For this review, use the dimensioned drawing (mm, ordinates from the lowest corner) and the shaded views. A direction names the side the tool comes from. Coordinates: 2 decimals unless noted, no trailing zeros. Loops run counter-clockwise (first coordinate to the right, second up) from the corner with the lowest first, then second, coordinate; pieces in that order, holes last. Notation, with made-up numbers: (73.25, -1) - (132.25, -1) arc R16 ccw to (132.25, 16) - close; hole circle Ø6 at (43.5, 32). An arc over 180 degrees is marked (long way). One line per item, written item: value. Start each with the question number.
1. We need section A-A, the plane z = 12. Give the boundary of the cut face in (x, y).
2. We need section D-D, the plane y = 12. Give the boundary of the cut face in (x, z).
3. For the marked faces 4 and 5, list the 3-axis set-ups (+Z, -Z, +X, -X, +Y, -Y) from which the entire face can be reached by the end or side of a thin tool; tool diameter is ignored.
4. Mouldability with a two-part tool opening along Y and no side actions: class the marked faces 1, 2 and 3 as +Y half, -Y half, draft (parallel to the pull), parting line (faces both ways), or undercut.
5. We need section C-C, the plane x = 8. Give the boundary of the cut face in (y, z), then the cut area to 3 significant figures.
6. Insertion check: P1, Ø7, axis at y = 23, z = 14, coming from the -X side; P2, Ø2, axis at y = 23.5, z = 4, coming from the -X side; P3, Ø7.5, axis at x = 20.5, y = 13.5, coming from the +Z side; P4, Ø8, axis at y = 12.5, z = 15.5, coming from the +X side. Each pin has a flat end and moves straight along its axis. Give the tip position at first contact, or say it passes through.
7. To check wall thickness, follow line 1 (X direction, y = 32, z = 21.5); line 2 (Z direction, x = 19.5, y = 13); line 3 (X direction, y = 27, z = 4.5). State the ranges of each line that lie inside material, in increasing order.
8. We need section B-B, the plane y = 24.5. Give the boundary of the cut face in (x, z).
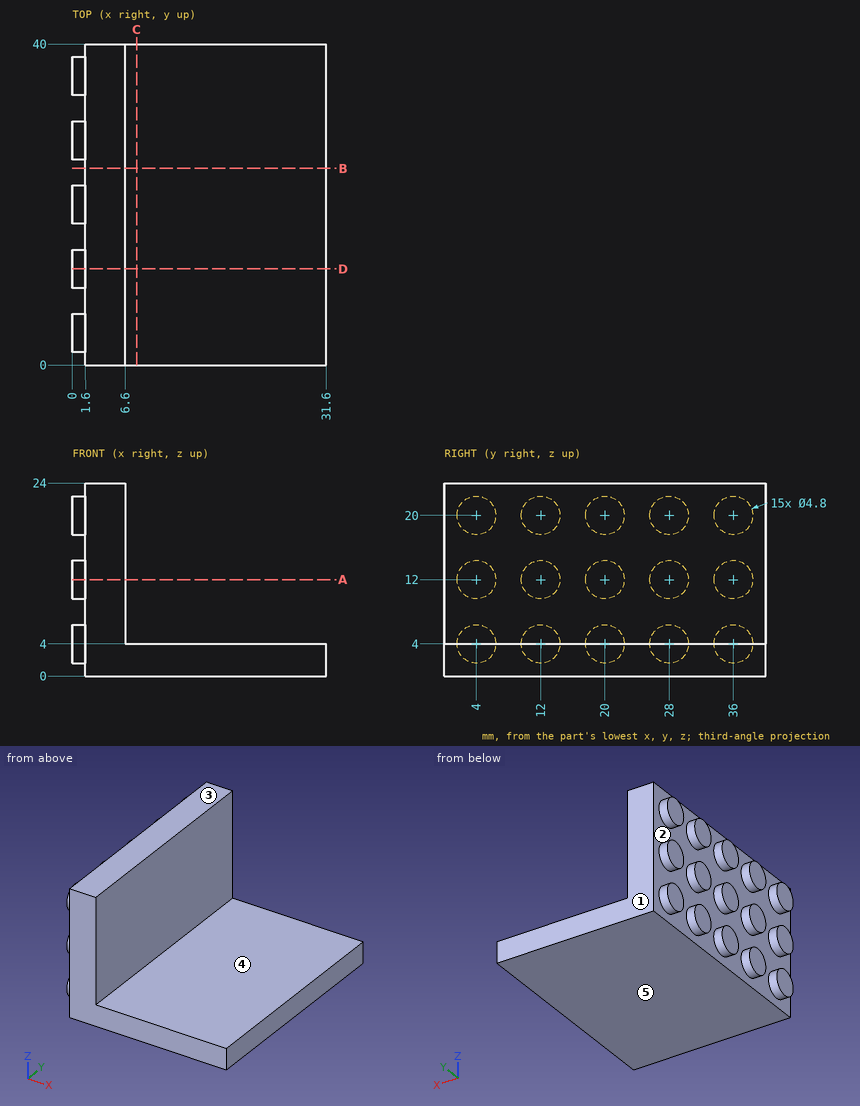
Findings below:
1. outline: (0, 1.6) - (1.6, 1.6) - (1.6, 0) - (6.6, 0) - (6.6, 40) - (1.6, 40) - (1.6, 38.4) - (0, 38.4) - (0, 33.6) - (1.6, 33.6) - (1.6, 30.4) - (0, 30.4) - (0, 25.6) - (1.6, 25.6) - (1.6, 22.4) - (0, 22.4) - (0, 17.6) - (1.6, 17.6) - (1.6, 14.4) - (0, 14.4) - (0, 9.6) - (1.6, 9.6) - (1.6, 6.4) - (0, 6.4) - close
2. outline: (0, 1.6) - (1.6, 1.6) - (1.6, 0) - (31.6, 0) - (31.6, 4) - (6.6, 4) - (6.6, 24) - (1.6, 24) - (1.6, 22.4) - (0, 22.4) - (0, 17.6) - (1.6, 17.6) - (1.6, 14.4) - (0, 14.4) - (0, 9.6) - (1.6, 9.6) - (1.6, 6.4) - (0, 6.4) - close
3. face 4: +Z, +X, +Y, -Y
3. face 5: -Z, +X, -X, +Y, -Y
4. face 1: +Y half
4. face 2: undercut
4. face 3: draft
5. outline: (0, 0) - (40, 0) - (40, 4) - (0, 4) - close
5. area: 160 mm2
6. P1: x = 0
6. P2: x = 1.6
6. P3: z = 4
6. P4: x = 6.6
7. line 1: 1.6 to 6.6
7. line 2: 0 to 4
7. line 3: 0 to 6.6
8. outline: (1.6, 0) - (31.6, 0) - (31.6, 4) - (6.6, 4) - (6.6, 24) - (1.6, 24) - close
